Check sheet for the modelled part. Datum: model origin and axes. Units: mm. A direction names the side the tool comes from. Coordinates: 2 decimals unless noted, no trailing zeros. Order: outer loops, then holes, each group sorted by start corner. A loop starts at its lowest first (then second) coordinate and runs counter-clockwise, first axis right, second up.
1. Set-up check for faces 4 (the flat face through (13, 0, -99)), 5 (the flat face through (68.901, -7.726, -98.6)): record each of +Z, -Z, +X, -X, +Y, -Y from which the full face is reachable in a straight line by a thin tool's end or side.
2. Gauge pin test, flat ends, axial feed: pin 1 Ø8 at (y, z) = (-4.5, -84) entering from -X; pin 2 Ø1 at (x, y) = (63, -7.5) entering from -Z. Record the tip position at first contact, or that the pin passes through.
3. Cross-section at A-A (x = 88.5). Enter the section's corners in (y, z), then the cut area to 3 significant figures.
4. Draft check along X on faces 1 (the flat face through (51, -12.5, -99)), 2 (the flat face through (99, -12.5, -99)), 3 (the flat face through (60, -15, -99)). Enter one of: released by +X, released by -X, zero draft, split by the parting line, or undercut.
5. Thickness scan on line 1 (X direction, y = -9.5, z = -81); line 2 (Y direction, x = 22.5, z = -168.5); line 3 (Y direction, x = 30, z = -66.5). Record the ranges inside material, lowest first.
```python
from build123d import *

# Parameters (mm, degrees)
BOSS_EXTRUDE1_DEPTH = 200


with BuildPart() as part:
    # Sketch1 → Boss-Extrude1 (new body)
    with BuildSketch(Plane.XY):
        with BuildLine():
            Line((0, -3.8), (0, -1))
            ThreePointArc((0, -1), (0.292893219, -0.292893219), (1, 0))
            Line((1, 0), (15, 0))
            Line((15, 0), (23.02057349, 0))
            Line((23.02057349, 0), (25.3, 0))
            Line((25.3, 0), (25.9, -0.75))
            Line((25.9, -0.75), (25.9, -2.5))
            Line((25.9, -2.5), (22, -2.5))
            Line((22, -2.5), (22, -5.5))
            Line((22, -5.5), (25.75, -9))
            Line((25.75, -9), (30, -9))
            Line((30, -9), (34.25, -9))
            Line((34.25, -9), (38, -5.5))
            Line((38, -5.5), (38, -2.5))
            Line((38, -2.5), (34.1, -2.5))
            Line((34.1, -2.5), (34.1, -0.75))
            Line((34.1, -0.75), (34.7, 0))
            Line((34.7, 0), (55.3, 0))
            Line((55.3, 0), (55.9, -0.75))
            Line((55.9, -0.75), (55.9, -2.5))
            Line((55.9, -2.5), (52, -2.5))
            Line((52, -2.5), (52, -5.5))
            Line((52, -5.5), (55.75, -9))
            Line((55.75, -9), (60, -9))
            Line((60, -9), (64.25, -9))
            Line((64.25, -9), (68, -5.5))
            Line((68, -5.5), (68, -2.5))
            Line((68, -2.5), (64.1, -2.5))
            Line((64.1, -2.5), (64.1, -0.75))
            Line((64.1, -0.75), (64.7, 0))
            Line((64.7, 0), (85.3, 0))
            Line((85.3, 0), (85.9, -0.75))
            Line((85.9, -0.75), (85.9, -2.5))
            Line((85.9, -2.5), (82, -2.5))
            Line((82, -2.5), (82, -5.5))
            Line((82, -5.5), (85.75, -9))
            Line((85.75, -9), (90, -9))
            Line((90, -9), (94.25, -9))
            Line((94.25, -9), (98, -5.5))
            Line((98, -5.5), (98, -2.5))
            Line((98, -2.5), (94.1, -2.5))
            Line((94.1, -2.5), (94.1, -0.75))
            Line((94.1, -0.75), (94.7, 0))
            Line((94.7, 0), (95.680089514, 0))
            Line((95.680089514, 0), (119, 0))
            ThreePointArc((119, 0), (119.707106781, -0.292893219), (120, -1))
            Line((120, -1), (120, -3.8))
            Line((120, -3.8), (118.5, -4.35))
            Line((118.5, -4.35), (118.5, -1.5))
            Line((118.5, -1.5), (116.5, -1.5))
            Line((116.5, -1.5), (115.25, -3))
            Line((115.25, -3), (115.25, -12))
            Line((115.25, -12), (116.5, -13.5))
            Line((116.5, -13.5), (118.5, -13.5))
            Line((118.5, -13.5), (118.5, -10.65))
            Line((118.5, -10.65), (120, -11.2))
            Line((120, -11.2), (120, -14))
            ThreePointArc((120, -14), (119.707106781, -14.707106781), (119, -15))
            Line((119, -15), (109.7, -15))
            Line((109.7, -15), (109.1, -14.25))
            Line((109.1, -14.25), (109.1, -12.5))
            Line((109.1, -12.5), (113, -12.5))
            Line((113, -12.5), (113, -9.5))
            Line((113, -9.5), (109.25, -6))
            Line((109.25, -6), (105, -6))
            Line((105, -6), (100.75, -6))
            Line((100.75, -6), (97, -9.5))
            Line((97, -9.5), (97, -12.5))
            Line((97, -12.5), (100.9, -12.5))
            Line((100.9, -12.5), (100.9, -14.25))
            Line((100.9, -14.25), (100.3, -15))
            Line((100.3, -15), (79.7, -15))
            Line((79.7, -15), (79.1, -14.25))
            Line((79.1, -14.25), (79.1, -12.5))
            Line((79.1, -12.5), (83, -12.5))
            Line((83, -12.5), (83, -9.5))
            Line((83, -9.5), (79.25, -6))
            Line((79.25, -6), (75, -6))
            Line((75, -6), (70.75, -6))
            Line((70.75, -6), (67, -9.5))
            Line((67, -9.5), (67, -12.5))
            Line((67, -12.5), (70.9, -12.5))
            Line((70.9, -12.5), (70.9, -14.25))
            Line((70.9, -14.25), (70.3, -15))
            Line((70.3, -15), (49.7, -15))
            Line((49.7, -15), (49.1, -14.25))
            Line((49.1, -14.25), (49.1, -12.5))
            Line((49.1, -12.5), (53, -12.5))
            Line((53, -12.5), (53, -9.5))
            Line((53, -9.5), (49.25, -6))
            Line((49.25, -6), (45, -6))
            Line((45, -6), (40.75, -6))
            Line((40.75, -6), (37, -9.5))
            Line((37, -9.5), (37, -12.5))
            Line((37, -12.5), (40.9, -12.5))
            Line((40.9, -12.5), (40.9, -14.25))
            Line((40.9, -14.25), (40.3, -15))
            Line((40.3, -15), (19.7, -15))
            Line((19.7, -15), (19.1, -14.25))
            Line((19.1, -14.25), (19.1, -12.5))
            Line((19.1, -12.5), (23, -12.5))
            Line((23, -12.5), (23, -9.5))
            Line((23, -9.5), (19.25, -6))
            Line((19.25, -6), (15, -6))
            Line((15, -6), (10.75, -6))
            Line((10.75, -6), (7, -9.5))
            Line((7, -9.5), (7, -12.5))
            Line((7, -12.5), (10.9, -12.5))
            Line((10.9, -12.5), (10.9, -14.25))
            Line((10.9, -14.25), (10.3, -15))
            Line((10.3, -15), (1, -15))
            ThreePointArc((1, -15), (0.292893219, -14.707106781), (0, -14))
            Line((0, -14), (0, -11.2))
            Line((0, -11.2), (1.5, -10.65))
            Line((1.5, -10.65), (1.5, -13.5))
            Line((1.5, -13.5), (3.5, -13.5))
            Line((3.5, -13.5), (4.75, -12))
            Line((4.75, -12), (4.75, -3))
            Line((4.75, -3), (3.5, -1.5))
            Line((3.5, -1.5), (1.5, -1.5))
            Line((1.5, -1.5), (1.5, -4.35))
            Line((1.5, -4.35), (0, -3.8))
        make_face()
    extrude(amount=-BOSS_EXTRUDE1_DEPTH)


solid = part.part
```
Data:
1. face 4: +Z, -Z, +X, -X, +Y
1. face 5: +Z, -Z
2. pin 1: stops at x = 0
2. pin 2: passes through
3. outline: (-15, -200) - (-9, -200) - (-9, 0) - (-15, 0) - close
3. area: 1,200 mm2
4. face 1: undercut
4. face 2: undercut
4. face 3: zero draft
5. line 1: x = 4.75 to 7, 23 to 37, 53 to 67, 83 to 97, 113 to 115.25
5. line 2: y = -15 to -12.5, -9.03 to -5.97, -2.5 to 0
5. line 3: y = -15 to -9
